Geometry check sheet. Reference: the model listing, model coordinates, mm. Round coordinates to 2 decimals unless told otherwise and drop trailing zeros. Write each loop counter-clockwise with the first axis right and the second up, starting at its lowest first coordinate (ties: lowest second). Pieces come first, ordered by that corner, then holes. Notation, with made-up numbers: (31.25, 31.25) -> (48.25, 31.25) arc R19 ccw to (48.25, 43.25) -> close; hole circle Ø5 at (65, 2.5). An arc over 180 degrees is marked (long way). Return JSON: item names as keys, results as strings. Group by question number.
from build123d import *

# Parameters (mm, degrees)
F1_DEPTH = 25
F2_R     = 5
F4_D     = 17.5


with BuildPart() as f1:
    # F0 (on Front) → F1 (new body)
    with BuildSketch(Plane.XZ):
        with BuildLine():
            Line((-33.945313, 0), (21.054687, 0))
            Line((21.054687, 0), (21.054687, 15))
            Line((21.054687, 15), (13.028848, 15))
            ThreePointArc((13.028848, 15), (3.028848, 5), (-6.971152, 15))
            Line((-6.971152, 15), (-33.945313, 15))
            Line((-33.945313, 15), (-33.945313, 0))
        make_face()
    extrude(amount=F1_DEPTH)

    # F2
    f2_edges = [f1.edges().sort_by_distance(p)[0] for p in [
        (-33.945313, -25, 7.5),
        (-33.945313, 0, 7.5),
    ]]
    fillet(f2_edges, radius=F2_R)

    # F4 (through all)
    with Locations(Plane.XY.offset(15)):
        with Locations((-22.615639, -12.5)):
            Hole(F4_D / 2)


solid = f1.part
1) Go/stop test with a flat-tipped pin: P1, Ø6, axis at x = 10, z = 9.5, coming from the +Y side. Record where the tip stops, or that it passes through.
2) Sectioned sample at C-C on x = -27.5. Enter the section's corners in (y, z).
3) Sectioned sample at D-D on z = 2.5. Enter the section's corners in (x, y).
4) Sectioned sample at A-A on y = -12.5. Enter the section's corners in (x, z).
5) Mould release check, pull along Y, two halves, no side actions. Record for faces 1 (the face through (-4, -25, 6)), 2 (the face through (-31, -10, 7)), 3 (the face through (3, -12, 5)): +Y half, -Y half, draft (parallel to the pull), parting line (faces both ways), or undercut.
6) Material ranges on probe 1 along Y at (x, z) = (-22.5, 13.5); probe 2 along X at (y, z) = (-17.5, 14.75); probe 3 along Z at (x, y) = (3.5, -14.5), recorded low to high. Write a range as [from, to].
7) Sectioned sample at B-B on z = 6.5. Enter the section's corners in (x, y).
Evaluation:
{
 "1": {"P1": "stops at y = 0"},
 "2": {"outline": "(-25, 0) -> (-19.76, 0) -> (-19.76, 15) -> (-25, 15) -> close; (-5.24, 0) -> (0, 0) -> (0, 15) -> (-5.24, 15) -> close"},
 "3": {"outline": "(-33.95, -20) arc R5 ccw to (-28.95, -25) -> (21.05, -25) -> (21.05, 0) -> (-28.95, 0) arc R5 ccw to (-33.95, -5) -> close; hole circle Ø17.5 at (-22.62, -12.5)"},
 "4": {"outline": "(-33.95, 0) -> (-31.37, 0) -> (-31.37, 15) -> (-33.95, 15) -> close; (-13.87, 0) -> (21.05, 0) -> (21.05, 15) -> (13.03, 15) arc R10 cw to (-6.97, 15) -> (-13.87, 15) -> close"},
 "5": {"face 1": "-Y half", "face 2": "undercut", "face 3": "draft"},
 "6": {"probe 1": "y = [-25, -21.25], [-3.75, 0]", "probe 2": "x = [-33.95, -29.8], [-15.43, -6.97], [13.03, 21.05]", "probe 3": "z = [0, 5.01]"},
 "7": {"outline": "(-33.95, -20) arc R5 ccw to (-28.95, -25) -> (-2.24, -25) -> (-2.24, 0) -> (-28.95, 0) arc R5 ccw to (-33.95, -5) -> close; (8.3, -25) -> (21.05, -25) -> (21.05, 0) -> (8.3, 0) -> close; hole circle Ø17.5 at (-22.62, -12.5)"}
}
